from build123d import *

# Parameters (mm, degrees)
F0_R     = 57
F0_R_2   = 53
F1_DEPTH = 13
F3_DEPTH = 4
F4_R     = 3
F5_R     = 54.8
F5_R_2   = 53
F6_DEPTH = 3


with BuildPart() as f1:
    # F0 (on Top) → F1 (new body)
    with BuildSketch(Plane.XY):
        Circle(F0_R)
        Circle(F0_R_2, mode=Mode.SUBTRACT)
    extrude(amount=F1_DEPTH)

    # F2 (on Top) → F3 (join)
    with BuildSketch(Plane.XY):
        with BuildLine():
            Line((-56.859476, 4), (-59.866518, 4))
            ThreePointArc((-59.866518, 4), (-60, 0), (-59.866518, -4))
            Line((-59.866518, -4), (-56.859476, -4))
            ThreePointArc((-56.859476, -4), (-57, 0), (-56.859476, 4))
        make_face()
        with BuildLine():
            ThreePointArc((4, 59.866518), (0, 60), (-4, 59.866518))
            Line((-4, 59.866518), (-4, 56.859476))
            ThreePointArc((-4, 56.859476), (0, 57), (4, 56.859476))
            Line((4, 56.859476), (4, 59.866518))
        make_face()
        with BuildLine():
            ThreePointArc((-4, -59.866518), (0, -60), (4, -59.866518))
            Line((4, -59.866518), (4, -56.859476))
            ThreePointArc((4, -56.859476), (0, -57), (-4, -56.859476))
            Line((-4, -56.859476), (-4, -59.866518))
        make_face()
        with BuildLine():
            Line((56.859476, -4), (59.866518, -4))
            ThreePointArc((59.866518, -4), (60, 0), (59.866518, 4))
            Line((59.866518, 4), (56.859476, 4))
            ThreePointArc((56.859476, 4), (57, 0), (56.859476, -4))
        make_face()
    extrude(amount=F3_DEPTH)

    # F4
    f4_edges = [f1.edges().sort_by_distance(p)[0] for p in [
        (59.866518, -4, 2),
        (59.866518, 4, 2),
        (-4, -59.866518, 2),
        (4, -59.866518, 2),
        (-59.866518, -4, 2),
        (-59.866518, 4, 2),
        (-4, 59.866518, 2),
        (4, 59.866518, 2),
    ]]
    fillet(f4_edges, radius=F4_R)

    # F5 (on face) → F6 (join)
    with BuildSketch(Plane.XY.offset(13)):
        Circle(F5_R)
        Circle(F5_R_2, mode=Mode.SUBTRACT)
    extrude(amount=F6_DEPTH)


solid = f1.part
Work out the finished part from the listing and answer in its coordinate system (mm). A direction names the side the tool comes from. Give positions to 0.01 mm unless a question says otherwise; leave off trailing zeros. Loops run counter-clockwise (first coordinate to the right, second up) from the corner with the lowest first, then second, coordinate; pieces in that order, holes last. Notation, with made-up numbers: (-34, 10) -> (-8, 10) arc R22 cw to (-8, 45) -> close; hole circle Ø4 at (-15.5, 61.25). An arc over 180 degrees is marked (long way). Use a Markdown table: item, result. Add a question column.
1) Which of the six approach directions +Z, -Z, +X, -X, +Y, -Y give full straight-line access (tool end or side, diameter ignored) to faces 1 (the cylindrical face through (-40.39, 37.036, 14.479)), 2 (the cylindrical face through (3.163, 59.07, 2.028))?
2) The part is cut by section A-A, the plane y = -16. Determine the outline of the cut face in (x, z).
3) For a pull along Y with two mould halves and no side action, classify faces 3 (the cylindrical face through (28, 45, 8)), 4 (the flat face through (35, -40, 0)), 5 (the cylindrical face through (52.654, -21.831, 6.409)) as +Y half, -Y half, draft (parallel to the pull), parting line (faces both ways), or undercut.
4) The part is cut by section B-B, the plane x = -13.5. Determine the outline of the cut face in (y, z).
5) The part is cut by section C-C, the plane z = 8.75. Determine the outline of the cut face in (x, y).
6) Consider line 1 along Y through (x, z) = (0, 3.75); line 2 along Y through (x, z) = (0, 9.5); line 3 along X through (y, z) = (35, 5.25). Determine where each line is inside the solid, lowest interval first.
7) Each of these flat-tipped pins is pushed along its axis until it touches: P1, Ø1.6, axis at x = 59, y = 1, coming from the +Z side; P2, Ø6, axis at y = -11.5, z = 6.5, coming from the -X side; P3, Ø1.5, axis at x = 21, z = 11, coming from the -Y side; P4, Ø8, axis at x = -41.5, y = -27.5, coming from the +Z side. Where does it stop, or does it pass through?
Reported:
| question | item | result |
|---|---|---|
| 1 | face 1 | +Z |
| 1 | face 2 | +Z, -Z, +X, +Y |
| 2 | outline | (-54.71, 0) -> (-50.53, 0) -> (-50.53, 16) -> (-52.41, 16) -> (-52.41, 13) -> (-54.71, 13) -> close; (50.53, 0) -> (54.71, 0) -> (54.71, 13) -> (52.41, 13) -> (52.41, 16) -> (50.53, 16) -> close |
| 3 | face 3 | undercut |
| 3 | face 4 | draft |
| 3 | face 5 | parting line |
| 4 | outline | (-55.38, 0) -> (-51.25, 0) -> (-51.25, 16) -> (-53.11, 16) -> (-53.11, 13) -> (-55.38, 13) -> close; (51.25, 0) -> (55.38, 0) -> (55.38, 13) -> (53.11, 13) -> (53.11, 16) -> (51.25, 16) -> close |
| 5 | outline | circle Ø114 at (0, 0); hole circle Ø106 at (0, 0) |
| 6 | line 1 | y = -60 to -53, 53 to 60 |
| 6 | line 2 | y = -57 to -53, 53 to 57 |
| 6 | line 3 | x = -44.99 to -39.8, 39.8 to 44.99 |
| 7 | P1 | stops at z = 4 |
| 7 | P2 | stops at x = -56.36 |
| 7 | P3 | stops at y = -53.28 |
| 7 | P4 | stops at z = 16 |
